from build123d import *

# Parameters (mm, degrees)
SKETCH1_W           = 15
SKETCH1_H           = 10
BOSS_EXTRUDE1_DEPTH = 57.5
SKETCH2_W           = 10.5
SKETCH2_H           = 5.5
BOSS_EXTRUDE2_DEPTH = 9.5


with BuildPart() as part:
    # Sketch1 → Boss-Extrude1 (new, symmetric)
    with BuildSketch(Plane(origin=(0, 0, 0), x_dir=(1, 0, 0), z_dir=(0, 1, 0))):
        Rectangle(SKETCH1_W, SKETCH1_H)
    extrude(amount=BOSS_EXTRUDE1_DEPTH, both=True)

    # Sketch2 → Boss-Extrude2 (add)
    with BuildSketch(Plane(origin=(0, 57.5, 0), x_dir=(1, 0, 0), z_dir=(0, 1, 0))):
        Rectangle(SKETCH2_W, SKETCH2_H)
    boss_extrude2 = extrude(amount=BOSS_EXTRUDE2_DEPTH)

    # Mirror1: Boss-Extrude2 across plane
    add(boss_extrude2.mirror(Plane.ZX))


solid = part.part
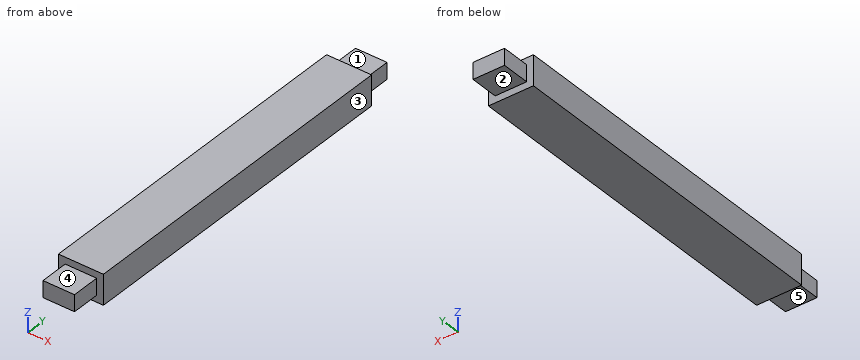
Here's how the part is built. I have some questions about the finished solid (model axes, mm). Face numbers are marked on the shaded views. A direction names the side the tool comes from. Coordinates: 2 decimals unless noted, no trailing zeros. Order: outer loops, then holes, each group sorted by start corner. A loop starts at its lowest first (then second) coordinate and runs counter-clockwise, first axis right, second up.
Item 1: If we section it at A-A on z = 1.5: List the corners of the cut face in (x, y) for me, plus the area to 3 significant figures.
Result sheet:
outline: (-7.5, -57.5) - (-5.25, -57.5) - (-5.25, -67) - (5.25, -67) - (5.25, -57.5) - (7.5, -57.5) - (7.5, 57.5) - (5.25, 57.5) - (5.25, 67) - (-5.25, 67) - (-5.25, 57.5) - (-7.5, 57.5) - close
area: 1,920 mm2
Item 2: For P1, Ø3, axis at y = 64.5, z = -0.5, coming from the -X side; P2, Ø3, axis at x = 0.5, y = 60.5, coming from the +Z side; P3, Ø6, axis at y = 63, z = 1, coming from the +X side, each with a flat end and sliding along its axis, tell me the tip position at first contact or that it passes through.
Result sheet:
P1: stops at x = -5.25
P2: stops at z = 2.75
P3: stops at x = 5.25
Item 3: If we section it at B-B on x = -2.5: List the corners of the cut face in (y, z) for me, plus the area to 3 significant figures.
Result sheet:
outline: (-67, -2.75) - (-57.5, -2.75) - (-57.5, -5) - (57.5, -5) - (57.5, -2.75) - (67, -2.75) - (67, 2.75) - (57.5, 2.75) - (57.5, 5) - (-57.5, 5) - (-57.5, 2.75) - (-67, 2.75) - close
area: 1,250 mm2
Item 4: I need wall thicknesses on line 1 (Y direction, x = -5, z = 3.5); line 2 (Z direction, x = -1.5, y = 60). Which ranges of each line are inside material? Lowest first, please.
Result sheet:
line 1: y = -57.5 to 57.5
line 2: z = -2.75 to 2.75
Item 5: For the marked faces 1, 2, 3, 4 and 5, which set-ups out of +Z, -Z, +X, -X, +Y, -Y let a thin tool reach every point of the face, with its end or its side?
Result sheet:
face 1: +Z, +X, -X, +Y
face 2: -Z, +X, -X, +Y
face 3: +Z, -Z, +X, +Y, -Y
face 4: +Z, +X, -X, -Y
face 5: -Z, +X, -X, -Y
